The listing builds one solid part. Answer for the finished solid, in the listing's coordinates (mm). Give positions to 0.01 mm unless a question says otherwise; leave off trailing zeros. Loops run counter-clockwise (first coordinate to the right, second up) from the corner with the lowest first, then second, coordinate; pieces in that order, holes last. Notation, with made-up numbers: (-22, -3.5) - (31, -3.5) arc R25 ccw to (31, 19.5) - close; hole circle Ø7 at (-3, 61.25). An arc over 180 degrees is marked (long way). Answer as CSV lines item,"result". Start each with the question number.
1) A cutting plane is placed at D-D (y = 0). Determine the outline of the cut face in (x, z), and give its area (3 significant figures).
2) A cutting plane is placed at B-B (z = 1.65). Determine the outline of the cut face in (x, y).
3) Find the intervals of material crossed by line 1 along Y through (x, z) = (4.5, 2.85); line 2 along X through (y, z) = (-1.25, 3.45); line 3 along X through (y, z) = (1.5, 3.45), in increasing order.
4) Flat-ended cylindrical pins translate along their axes: pin 1 (1.5 mm diameter, centred on x = 3.5, y = 1, fed in from +Z); pin 2 (2 mm diameter, centred on y = -1.5, z = 3.5, fed in from -X). Find the tip coordinate at first contact, or state that the pin passes through.
5) A cutting plane is placed at C-C (y = 3.3). Determine the outline of the cut face in (x, z), and give its area (3 significant figures).
6) A cutting plane is placed at A-A (x = 4.5). Determine the outline of the cut face in (y, z), and give its area (3 significant figures).
7) For a pull along Y with two mould halves and no side action, classify faces 1 (the face through (10, 3, 2)), 2 (the face through (2.85, 0.07, 1.97)), 3 (the face through (0, -3, 2)) as pulls with the +Y half, pulls with the -Y half, needs draft (parallel to the pull), parting line crosses it, or undercut.
```python
from build123d import *

# Parameters (mm, degrees)
SKETCH1_W           = 20
SKETCH1_H           = 7
SKETCH1_R           = 1.65
BOSS_EXTRUDE1_DEPTH = 4
BOSS_EXTRUDE2_DEPTH = 0.2
FILLET1_R           = 5


with BuildPart() as part:
    # Sketch1 → Boss-Extrude1 (new body)
    with BuildSketch(Plane.XY):
        with Locations((0, 0.5)):
            Rectangle(SKETCH1_W, SKETCH1_H)
        with Locations((-4.5, 0)):
            Circle(SKETCH1_R, mode=Mode.SUBTRACT)
        with Locations((4.5, 0)):
            Circle(SKETCH1_R, mode=Mode.SUBTRACT)
    extrude(amount=BOSS_EXTRUDE1_DEPTH)

    # Sketch2 → Boss-Extrude2 (add)
    with BuildSketch(Plane.XY.offset(4)):
        with BuildLine():
            Line((-3, 3.5), (3, 3.5))
            ThreePointArc((3, 3.5), (3.2, 3.3), (3, 3.1))
            Line((3, 3.1), (-3, 3.1))
            ThreePointArc((-3, 3.1), (-3.2, 3.3), (-3, 3.5))
        make_face()
    extrude(amount=BOSS_EXTRUDE2_DEPTH)

    # Fillet1
    fillet1_edges = [part.edges().sort_by_distance(p)[0] for p in [
        (10, -3, 2),
        (-10, -3, 2),
    ]]
    fillet(fillet1_edges, radius=FILLET1_R)


solid = part.part
```
Ans:
1,outline,"(-9.58, 0) - (-6.15, 0) - (-6.15, 4) - (-9.58, 4) - close; (-2.85, 0) - (2.85, 0) - (2.85, 4) - (-2.85, 4) - close; (6.15, 0) - (9.58, 0) - (9.58, 4) - (6.15, 4) - close"
1,area,"50.3 mm2"
2,outline,"(-10, 2) arc R5 ccw to (-5, -3) - (5, -3) arc R5 ccw to (10, 2) - (10, 4) - (-10, 4) - close; hole circle Ø3.3 at (-4.5, 0); hole circle Ø3.3 at (4.5, 0)"
3,line 1,"-3 to -1.65, 1.65 to 4"
3,line 2,"-8.8 to -5.58, -3.42 to 3.42, 5.58 to 8.8"
3,line 3,"-9.97 to -5.19, -3.81 to 3.81, 5.19 to 9.97"
4,pin 1,"z = 4"
4,pin 2,"x = -9.33"
5,outline,"(-10, 0) - (10, 0) - (10, 4) - (3.2, 4) - (3.2, 4.2) - (-3.2, 4.2) - (-3.2, 4) - (-10, 4) - close"
5,area,"81.3 mm2"
6,outline,"(-3, 0) - (-1.65, 0) - (-1.65, 4) - (-3, 4) - close; (1.65, 0) - (4, 0) - (4, 4) - (1.65, 4) - close"
6,area,"14.8 mm2"
7,face 1,"needs draft"
7,face 2,"undercut"
7,face 3,"pulls with the -Y half"
